Model file for the job. Use its own axes, mm. A direction names the side the tool comes from. Give positions to 0.01 mm unless a question says otherwise; leave off trailing zeros. Order: outer loops, then holes, each group sorted by start corner. A loop starts at its lowest first (then second) coordinate and runs counter-clockwise, first axis right, second up. Notation, with made-up numbers: M -16.75,62 L -10.75,62 A12 ccw -10.75,70 Z; hole C 80,24 d5. An arc over 180 degrees is marked long. Return JSON: item names as keys, results as strings. Group by question number.
1. Pin check, flat tips, straight feed: pin 1 (2.5 mm diameter, centred on x = -35, z = 16.5, fed in from +Y); pin 2 (2.5 mm diameter, centred on x = 13.93, y = 5, fed in from +Z); pin 3 (2 mm diameter, centred on x = 8.43, z = 20.98, fed in from -Y); pin 4 (1.3 mm diameter, centred on x = -20.5, z = -10, fed in from -Y). Stop position of each tip, or through.
2. Slice it at C-C on x = -14. List the corners of the cut face in (y, z).
3. Two-plate mould, pull along Z, no slides. Class faces 6 (the face through (-24.55, 4.37, 31.91)), 7 (the face through (8, 7.75, 21)), 8 (the face through (-26, 5, -17.421)): released by +Z, released by -Z, zero draft, split by the parting line, or undercut.
4. Slice it at A-A on y = 8.5. List the corners of the cut face in (x, z), then the cut area to 3 significant figures.
5. 3-axis set-ups, long thin cutter, end or side, ignore diameter. For faces 1 (the face through (-35, 7, -5)), 2 (the face through (7.356, 8.859, -9.843)), 3 (the face through (-24.5, 4.5, -19.9)), 4 (the face through (-21, 7.75, 20)), 5 (the face through (14, 5, 29.379)): which of +Z, -Z, +X, -X, +Y, -Y reach the whole face in a straight line?
6. Slice it at D-D on y = 5. List the corners of the cut face in (x, z), then the cut area to 3 significant figures.
7. Wall check: probe 1 along X at (y, z) = (5, -18); probe 2 along Z at (x, y) = (18, 9); probe 3 along X at (y, z) = (5.75, 31). Give the ranges that are in metal, low to high. Write a range as [from, to].
8. Slice it at B-B on y = 1.5. List the corners of the cut face in (x, z), then the cut area to 3 significant figures.
from build123d import *
from build123d.topology import SkipClean

# Parameters (mm, degrees)
EXTRUDE_3_DEPTH     = 7
EXTRUDE_4_DEPTH     = 0.75
EXTRUDE_5_DEPTH     = 0.75
EXTRUDE_6_DEPTH     = 2.25
EXTRUDE_7_DEPTH     = 2.25
SKETCH_8_R          = 1.65
CUT_EXTRUDE_1_DEPTH = 5
CUT_EXTRUDE_START   = -5
SKETCH_9_R          = 1.65
CUT_EXTRUDE_2_DEPTH = 5


with BuildPart() as part:
    # Sketch 1 → Extrude 3 (new body)
    with BuildSketch(Plane(origin=(0, 0, 0), x_dir=(1, 0, 0), z_dir=(0, 1, 0))):
        with BuildLine():
            Line((-36.072982456, 22.421052632), (-36.072982456, 3.819011603))
            ThreePointArc((-36.072982456, 3.819011603), (-35.719367467, 3.340920159), (-35.158696742, 3.539069918))
            ThreePointArc((-35.158696742, 3.539069918), (-31.213626847, 7.665367614), (-26.125018269, 10.253025221))
            ThreePointArc((-26.125018269, 10.253025221), (-25.960902102, 10.314118117), (-25.79025857, 10.353453131))
            ThreePointArc((-25.79025857, 10.353453131), (-19.301572904, 10.928509809), (-13.072982456, 9.021052632))
            ThreePointArc((-13.072982456, 9.021052632), (-5.321033393, -12.372389376), (-25.79025857, -22.311347868))
            ThreePointArc((-25.79025857, -22.311347868), (-25.960902102, -22.272012853), (-26.125018269, -22.210919958))
            ThreePointArc((-26.125018269, -22.210919958), (-31.213626847, -19.623262351), (-35.158696742, -15.496964655))
            ThreePointArc((-35.158696742, -15.496964655), (-35.719367467, -15.298814896), (-36.072982456, -15.77690634))
            Line((-36.072982456, -15.77690634), (-36.072982456, -34.378947368))
            Line((-36.072982456, -34.378947368), (23.927017544, -34.378947368))
            Line((23.927017544, -34.378947368), (23.927017544, 22.421052632))
            Line((23.927017544, 22.421052632), (-36.072982456, 22.421052632))
        make_face()
    extrude(amount=EXTRUDE_3_DEPTH)

    # Sketch 5 → Extrude 4 (add)
    with BuildSketch(Plane(origin=(0, 7, 0), x_dir=(1, 0, 0), z_dir=(0, 1, 0))):
        with BuildLine():
            Line((-36.072982456, -34.378947368), (23.927017544, -34.378947368))
            Line((23.927017544, -34.378947368), (23.927017544, -18.478947368))
            Line((23.927017544, -18.478947368), (-9.551263834, -18.478947368))
            ThreePointArc((-9.551263834, -18.478947368), (-17.168250345, -22.524432165), (-25.79025857, -22.311347868))
            ThreePointArc((-25.79025857, -22.311347868), (-25.960902102, -22.272012853), (-26.125018269, -22.210919958))
            ThreePointArc((-26.125018269, -22.210919958), (-29.567347581, -20.704631092), (-32.594701078, -18.478947368))
            Line((-32.594701078, -18.478947368), (-36.072982456, -18.478947368))
            Line((-36.072982456, -18.478947368), (-36.072982456, -34.378947368))
        make_face()
    extrude(amount=EXTRUDE_4_DEPTH)

    # Sketch 5_3 → Extrude 5 (add)
    with BuildSketch(Plane(origin=(0, 7, 0), x_dir=(1, 0, 0), z_dir=(0, 1, 0))):
        with BuildLine():
            Line((-9.551263834, 6.521052632), (23.927017544, 6.521052632))
            Line((23.927017544, 6.521052632), (23.927017544, 22.421052632))
            Line((23.927017544, 22.421052632), (-36.072982456, 22.421052632))
            Line((-36.072982456, 22.421052632), (-36.072982456, 6.521052632))
            Line((-36.072982456, 6.521052632), (-32.594701078, 6.521052632))
            ThreePointArc((-32.594701078, 6.521052632), (-29.567347581, 8.746736355), (-26.125018269, 10.253025221))
            ThreePointArc((-26.125018269, 10.253025221), (-25.960902102, 10.314118117), (-25.79025857, 10.353453131))
            ThreePointArc((-25.79025857, 10.353453131), (-17.168250345, 10.566537428), (-9.551263834, 6.521052632))
        make_face()
    extrude(amount=EXTRUDE_5_DEPTH)

    # Sketch 6 → Extrude 6 (add)
    with BuildSketch(Plane(origin=(0, 7.75, 0), x_dir=(1, 0, 0), z_dir=(0, 1, 0))):
        with BuildLine():
            Line((-36.072982456, -34.378947368), (23.927017544, -34.378947368))
            Line((23.927017544, -34.378947368), (23.927017544, -20.978947368))
            Line((23.927017544, -20.978947368), (9.777017544, -20.978947368))
            ThreePointArc((9.777017544, -20.978947368), (8.427017544, -22.328947368), (7.077017544, -20.978947368))
            Line((7.077017544, -20.978947368), (-7.222982456, -20.978947368))
            ThreePointArc((-7.222982456, -20.978947368), (-8.572982456, -22.328947368), (-9.922982456, -20.978947368))
            Line((-9.922982456, -20.978947368), (-13.072982456, -20.978947368))
            ThreePointArc((-13.072982456, -20.978947368), (-19.301572904, -22.886404546), (-25.79025857, -22.311347868))
            ThreePointArc((-25.79025857, -22.311347868), (-25.960902102, -22.272012853), (-26.125018269, -22.210919958))
            ThreePointArc((-26.125018269, -22.210919958), (-29.567347581, -20.704631092), (-32.594701078, -18.478947368))
            Line((-32.594701078, -18.478947368), (-36.072982456, -18.478947368))
            Line((-36.072982456, -18.478947368), (-36.072982456, -34.378947368))
        make_face()
        with BuildLine():
            ThreePointArc((-25.79025857, -22.311347868), (-19.301572904, -22.886404546), (-13.072982456, -20.978947368))
            Line((-13.072982456, -20.978947368), (-24.222982456, -20.978947368))
            ThreePointArc((-24.222982456, -20.978947368), (-24.698574872, -22.007495557), (-25.79025857, -22.311347868))
        make_face()
        with BuildLine():
            ThreePointArc((-13.072982456, -20.978947368), (-11.232409582, -19.841238864), (-9.551263834, -18.478947368))
            Line((-9.551263834, -18.478947368), (-32.594701078, -18.478947368))
            ThreePointArc((-32.594701078, -18.478947368), (-29.567347581, -20.704631092), (-26.125018269, -22.210919958))
            ThreePointArc((-26.125018269, -22.210919958), (-26.306893776, -19.845865653), (-24.222982456, -20.978947368))
            Line((-24.222982456, -20.978947368), (-13.072982456, -20.978947368))
        make_face()
        with BuildLine():
            Line((9.777017544, -20.978947368), (23.927017544, -20.978947368))
            Line((23.927017544, -20.978947368), (23.927017544, -18.478947368))
            Line((23.927017544, -18.478947368), (-9.551263834, -18.478947368))
            ThreePointArc((-9.551263834, -18.478947368), (-11.232409582, -19.841238864), (-13.072982456, -20.978947368))
            Line((-13.072982456, -20.978947368), (-9.922982456, -20.978947368))
            ThreePointArc((-9.922982456, -20.978947368), (-8.572982456, -19.628947368), (-7.222982456, -20.978947368))
            Line((-7.222982456, -20.978947368), (7.077017544, -20.978947368))
            ThreePointArc((7.077017544, -20.978947368), (8.427017544, -19.628947368), (9.777017544, -20.978947368))
        make_face()
    extrude(amount=EXTRUDE_6_DEPTH)

    # Sketch 7 → Extrude 7 (add)
    with BuildSketch(Plane(origin=(0, 7.75, 0), x_dir=(1, 0, 0), z_dir=(0, 1, 0))):
        with BuildLine():
            Line((23.927017544, 9.021052632), (23.927017544, 22.421052632))
            Line((23.927017544, 22.421052632), (-36.072982456, 22.421052632))
            Line((-36.072982456, 22.421052632), (-36.072982456, 6.521052632))
            Line((-36.072982456, 6.521052632), (-32.594701078, 6.521052632))
            ThreePointArc((-32.594701078, 6.521052632), (-29.567347581, 8.746736355), (-26.125018269, 10.253025221))
            ThreePointArc((-26.125018269, 10.253025221), (-25.960902102, 10.314118117), (-25.79025857, 10.353453131))
            ThreePointArc((-25.79025857, 10.353453131), (-19.301572904, 10.928509809), (-13.072982456, 9.021052632))
            Line((-13.072982456, 9.021052632), (-9.922982456, 9.021052632))
            ThreePointArc((-9.922982456, 9.021052632), (-8.572982456, 10.371052632), (-7.222982456, 9.021052632))
            Line((-7.222982456, 9.021052632), (7.077017544, 9.021052632))
            ThreePointArc((7.077017544, 9.021052632), (8.427017544, 10.371052632), (9.777017544, 9.021052632))
            Line((9.777017544, 9.021052632), (23.927017544, 9.021052632))
        make_face()
        with BuildLine():
            Line((-32.594701078, 6.521052632), (-9.551263834, 6.521052632))
            ThreePointArc((-9.551263834, 6.521052632), (-11.232409582, 7.883344127), (-13.072982456, 9.021052632))
            Line((-13.072982456, 9.021052632), (-24.222982456, 9.021052632))
            ThreePointArc((-24.222982456, 9.021052632), (-26.306893776, 7.887970916), (-26.125018269, 10.253025221))
            ThreePointArc((-26.125018269, 10.253025221), (-29.567347581, 8.746736355), (-32.594701078, 6.521052632))
        make_face()
        with BuildLine():
            Line((-24.222982456, 9.021052632), (-13.072982456, 9.021052632))
            ThreePointArc((-13.072982456, 9.021052632), (-19.301572904, 10.928509809), (-25.79025857, 10.353453131))
            ThreePointArc((-25.79025857, 10.353453131), (-24.698574872, 10.04960082), (-24.222982456, 9.021052632))
        make_face()
        with BuildLine():
            Line((23.927017544, 6.521052632), (23.927017544, 9.021052632))
            Line((23.927017544, 9.021052632), (9.777017544, 9.021052632))
            ThreePointArc((9.777017544, 9.021052632), (8.427017544, 7.671052632), (7.077017544, 9.021052632))
            Line((7.077017544, 9.021052632), (-7.222982456, 9.021052632))
            ThreePointArc((-7.222982456, 9.021052632), (-8.572982456, 7.671052632), (-9.922982456, 9.021052632))
            Line((-9.922982456, 9.021052632), (-13.072982456, 9.021052632))
            ThreePointArc((-13.072982456, 9.021052632), (-11.232409582, 7.883344127), (-9.551263834, 6.521052632))
            Line((-9.551263834, 6.521052632), (23.927017544, 6.521052632))
        make_face()
    extrude(amount=EXTRUDE_7_DEPTH)

    # Sketch 8 → Cut-Extrude 1 (cut)
    with SkipClean():  # the faces are left unmerged after this step: merging them gives an invalid solid
        with BuildSketch(Plane.XY.offset(34.378947368)):
            with Locations((-26.072982456, 5)):
                Circle(SKETCH_8_R)
            with Locations((13.927017544, 5)):
                Circle(SKETCH_8_R)
        extrude(amount=-CUT_EXTRUDE_1_DEPTH, mode=Mode.SUBTRACT)

    # Sketch 9 → Cut-Extrude 2 (cut)
    with SkipClean():  # the faces are left unmerged after this step: merging them gives an invalid solid
        with BuildSketch(Plane(origin=(0, 0, -22.421052632), x_dir=(-1, 0, 0), z_dir=(0, 0, -1)).offset(CUT_EXTRUDE_START)):
            with Locations(Location((26.072982456, 5, 0), (0, 0, 180))):
                Circle(SKETCH_9_R)
            with Locations(Location((-13.927017544, 5, 0), (0, 0, 180))):
                Circle(SKETCH_9_R)
        extrude(amount=CUT_EXTRUDE_2_DEPTH, mode=Mode.SUBTRACT)


solid = part.part
Result:
{
 "1": {"pin 1": "stops at y = 7", "pin 2": "stops at z = 29.38", "pin 3": "stops at y = 0", "pin 4": "stops at y = 7.75"},
 "2": {"outline": "M 0,-22.42 L 10,-22.42 L 10,-6.52 L 7.75,-6.52 L 7.75,-9.48 L 0,-9.48 Z; M 0,21.44 L 7.75,21.44 L 7.75,18.48 L 10,18.48 L 10,34.38 L 0,34.38 Z"},
 "3": {"face 6": "zero draft", "face 7": "undercut", "face 8": "released by -Z"},
 "4": {"outline": "M -36.07,-22.42 L 23.93,-22.42 L 23.93,-6.52 L -36.07,-6.52 Z; M -36.07,18.48 L 23.93,18.48 L 23.93,34.38 L -36.07,34.38 Z; hole C -25.57,-9.02 d2.7; hole C -25.57,20.98 d2.7; hole C -8.57,-9.02 d2.7; hole C -8.57,20.98 d2.7; hole C 8.43,-9.02 d2.7; hole C 8.43,20.98 d2.7", "area": "1,870 mm2"},
 "5": {"face 1": "+X, -X, +Y", "face 2": "+Y", "face 3": "-Z", "face 4": "-Y", "face 5": "+Z"},
 "6": {"outline": "M -36.07,-22.42 L -27.72,-22.42 L -27.72,-17.42 L -24.42,-17.42 L -24.42,-22.42 L 12.28,-22.42 L 12.28,-17.42 L 15.58,-17.42 L 15.58,-22.42 L 23.93,-22.42 L 23.93,34.38 L 15.58,34.38 L 15.58,29.38 L 12.28,29.38 L 12.28,34.38 L -24.42,34.38 L -24.42,29.38 L -27.72,29.38 L -27.72,34.38 L -36.07,34.38 L -36.07,15.78 A0.5 ccw -35.16,15.5 A17 cw -26.13,22.21 A1.35 cw -25.79,22.31 A17 cw long -25.79,-10.35 A1.35 cw -26.13,-10.25 A17 cw -35.16,-3.54 A0.5 ccw -36.07,-3.82 Z", "area": "2,450 mm2"},
 "7": {"probe 1": "x = [-36.07, -27.72], [-24.42, 12.28], [15.58, 23.93]", "probe 2": "z = [-22.42, -6.52], [18.48, 34.38]", "probe 3": "x = [-36.07, -27.54], [-24.6, 12.46], [15.4, 23.93]"},
 "8": {"outline": "M -36.07,-22.42 L 23.93,-22.42 L 23.93,34.38 L -36.07,34.38 L -36.07,15.78 A0.5 ccw -35.16,15.5 A17 cw -26.13,22.21 A1.35 cw -25.79,22.31 A17 cw long -25.79,-10.35 A1.35 cw -26.13,-10.25 A17 cw -35.16,-3.54 A0.5 ccw -36.07,-3.82 Z", "area": "2,520 mm2"}
}
